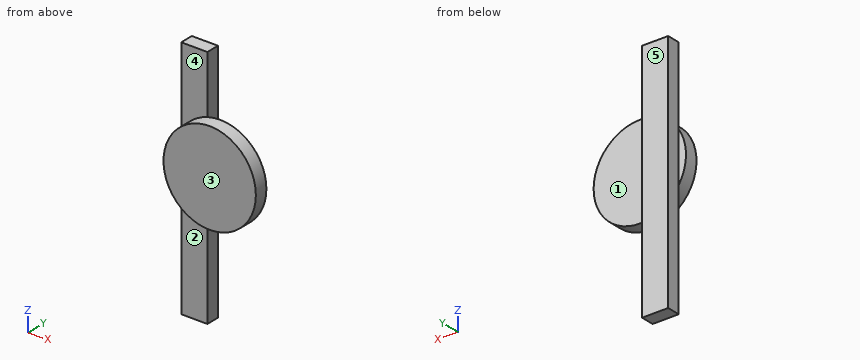
```python
from build123d import *

# Parameters (mm, degrees)
F0_R     = 87.939634
F1_DEPTH = 25.4
F2_W     = 49.783926
F2_H     = 460.88621
F3_DEPTH = 25.4


with BuildPart() as f1:
    # F0 (on Front) → F1 (new body)
    with BuildSketch(Plane.XZ):
        Circle(F0_R)
    extrude(amount=F1_DEPTH)

    # F2 (on face) → F3 (join)
    with BuildSketch(Plane(origin=(0, 0, 0), x_dir=(-1, 0, 0), z_dir=(0, 1, 0))):
        with BuildLine():
            Line((74.138304, 194.744006), (24.354378, 194.744006))
            Line((24.354378, 194.744006), (24.354378, 84.499962))
            ThreePointArc((24.354378, 84.499962), (52.642567, 70.442454), (74.138304, 47.295783))
            Line((74.138304, 47.295783), (74.138304, 194.744006))
        make_face()
        with BuildLine():
            ThreePointArc((74.138304, -47.295783), (52.642567, -70.442454), (24.354378, -84.499962))
            Line((24.354378, -84.499962), (24.354378, -266.142204))
            Line((24.354378, -266.142204), (74.138304, -266.142204))
            Line((74.138304, -266.142204), (74.138304, -47.295783))
        make_face()
        with Locations((49.246341, -35.699099)):
            Rectangle(F2_W, F2_H)
    extrude(amount=F3_DEPTH)


solid = f1.part
```
Build history of the part. All positions in model axes, mm. Face numbers are marked on the shaded views. A direction names the side the tool comes from. Give positions to 0.01 mm unless a question says otherwise; leave off trailing zeros. Loops run counter-clockwise (first coordinate to the right, second up) from the corner with the lowest first, then second, coordinate; pieces in that order, holes last. Notation, with made-up numbers: (-35, 6.25) - (22, 6.25) arc R9 cw to (22, 17.25) - close; hole circle Ø8 at (-31, 39.5). An arc over 180 degrees is marked (long way). Use a Markdown table: item, result.
(1) Band-saw the part on B-B (x = -32). Give the cut face in (y, z), and give its area (3 significant figures).
Taken from the geometry:
| item | result |
|---|---|
| outline | (-25.4, -81.91) - (0, -81.91) - (0, -266.14) - (25.4, -266.14) - (25.4, 194.74) - (0, 194.74) - (0, 81.91) - (-25.4, 81.91) - close |
| area | 15,900 mm2 |
(2) Band-saw the part on D-D (z = 143.5). Give the cut face in (x, y), and give its area (3 significant figures).
Taken from the geometry:
| item | result |
|---|---|
| outline | (-74.14, 0) - (-24.35, 0) - (-24.35, 25.4) - (-74.14, 25.4) - close |
| area | 1,260 mm2 |
(3) Wall check: line 1 along X through (y, z) = (13.5, 69.5); line 2 along Y through (x, z) = (34, -38.5); line 3 along Y through (x, z) = (-58, 139). Give the ranges that are in metal, low to high.
Taken from the geometry:
| item | result |
|---|---|
| line 1 | -74.14 to -24.35 |
| line 2 | -25.4 to 0 |
| line 3 | 0 to 25.4 |
(4) Pull direction Y, two halves, no side cores. Call the marked faces 4 and 5: +Y half, -Y half, draft (parallel to the pull), parting line (faces both ways), or undercut.
Taken from the geometry:
| item | result |
|---|---|
| face 4 | -Y half |
| face 5 | +Y half |
(5) Which spindle directions (+Z, -Z, +X, -X, +Y, -Y) get a long thin tool onto all of the face, cutting with end or side? Do the marked faces 1, 2 and 3. Say none if no direction does.
Taken from the geometry:
| item | result |
|---|---|
| face 1 | +Z, -Z, +X, +Y |
| face 2 | -Z, -X, -Y |
| face 3 | +Z, -Z, +X, -X, -Y |
(6) Drop flat-ended pins along their axis: pin 1 Ø5 at (y, z) = (-15, 56) entering from +X; pin 2 Ø6 at (x, y) = (-1, -12.5) entering from -Z; pin 3 Ø3 at (y, z) = (2, 36) entering from -X; pin 4 Ø15 at (x, z) = (-80.5, -7) entering from +Y. Give the stop position or say it passes through.
Taken from the geometry:
| item | result |
|---|---|
| pin 1 | x = 69.79 |
| pin 2 | z = -87.94 |
| pin 3 | x = -74.14 |
| pin 4 | y = 25.4 |
(7) Band-saw the part on C-C (y = 17). Give the cut face in (x, z).
Taken from the geometry:
| item | result |
|---|---|
| outline | (-74.14, -266.14) - (-24.35, -266.14) - (-24.35, 194.74) - (-74.14, 194.74) - close |
(8) Band-saw the part on A-A (z = 0). Give the cut face in (x, y).
Taken from the geometry:
| item | result |
|---|---|
| outline | (-87.94, -25.4) - (87.94, -25.4) - (87.94, 0) - (-24.35, 0) - (-24.35, 25.4) - (-74.14, 25.4) - (-74.14, 0) - (-87.94, 0) - close |
